Can you work these out from the model? Positions are in its coordinate system, mm. A direction names the side the tool comes from. Coordinates: 2 decimals unless noted, no trailing zeros. Write each loop counter-clockwise with the first axis right and the second up, starting at its lowest first coordinate (ties: lowest second). Pieces come first, ordered by that corner, then holes. Notation, with made-up numbers: M -36,1 L -3,1 A15 ccw -3,5 Z; hole C 70,-20.5 d8. An arc over 180 degrees is marked long. Use one line per item in the form item = value. Start each with the question number.
```python
from build123d import *

# Parameters (mm, degrees)
FILLET1_R                       = 2
BOSS_EXTRUDE1_REACH             = 54.062
SKETCH2_R                       = 1.5
BOSS_EXTRUDE1_DIRECTION_2_REACH = 54.062
CHAMFER1_SIZE                   = 1
CUT_EXTRUDE1_START              = -3
CUT_EXTRUDE1_DEPTH              = 3


with BuildPart() as part:
    # Sketch1 → Revolve1 (revolve)
    with BuildSketch(Plane.XY):
        Polygon((17.7, 0), (17.7, 3.5), (0, 28.778219719), (0, 43.98066929), (3, 43.98066929), (3, 27.98066929), (19.7, 4.130597578), (19.7, 0), align=None)
    revolve(axis=Axis((0, 0, 0), (0, 1, 0)))

    # Fillet1
    fillet1_edges = [part.edges().sort_by_distance(p)[0] for p in [
        (-3, 27.98066929, 0),
        (-19.7, 4.130597578, 0),
    ]]
    fillet(fillet1_edges, radius=FILLET1_R)

    # Boss-Extrude1: up to this cone (the profile starts inside it)
    boss_extrude1_end = Plane(origin=(0, 12, 0), z_dir=(0, -1, 0)).offset(-16.778218719) * Cone(1e-06, 58.179162981, 83.088454645, align=(Align.CENTER, Align.CENTER, Align.MIN), mode=Mode.PRIVATE)
    # Sketch2 → Boss-Extrude1 (add, up to the surface)
    with BuildSketch(Plane(origin=(0, 0, 0), x_dir=(0, 0, -1), z_dir=(1, 0, 0)), mode=Mode.PRIVATE) as boss_extrude1_sk1:
        with Locations(Location((0, 12, 0), (0, 0, 356.704943747))):
            Circle(SKETCH2_R)
    boss_extrude1_tool1 = extrude(boss_extrude1_sk1.sketch, amount=BOSS_EXTRUDE1_REACH, mode=Mode.PRIVATE) & boss_extrude1_end
    add(boss_extrude1_tool1.solids().sort_by_distance((0, 12, 0))[0])

    # Boss-Extrude1 direction 2: up to this cone (the profile starts inside it)
    boss_extrude1_direction_2_end = Plane(origin=(0, 12, 0), z_dir=(0, -1, 0)).offset(-16.778218719) * Cone(1e-06, 58.179162981, 83.088454645, align=(Align.CENTER, Align.CENTER, Align.MIN), mode=Mode.PRIVATE)
    # Sketch2 → Boss-Extrude1 direction 2 (add, up to the surface)
    with BuildSketch(Plane(origin=(0, 0, 0), x_dir=(0, 0, -1), z_dir=(1, 0, 0)), mode=Mode.PRIVATE) as boss_extrude1_direction_2_sk1:
        with Locations(Location((0, 12, 0), (0, 0, 356.704943747))):
            Circle(SKETCH2_R)
    boss_extrude1_direction_2_tool1 = extrude(boss_extrude1_direction_2_sk1.sketch, amount=-BOSS_EXTRUDE1_DIRECTION_2_REACH, mode=Mode.PRIVATE) & boss_extrude1_direction_2_end
    add(boss_extrude1_direction_2_tool1.solids().sort_by_distance((0, 12, 0))[0])

    # Chamfer1
    chamfer1_edges = [part.edges().sort_by_distance(p)[0] for p in [
        (-3, 43.98066929, 0),
    ]]
    chamfer(chamfer1_edges, length=CHAMFER1_SIZE)

    # Sketch3 → Cut-Extrude1 (cut)
    with BuildSketch(Plane.XZ.offset(CUT_EXTRUDE1_START)):
        with BuildLine():
            Line((-3.2, 18.627130751), (-3.2, 17.408331339))
            ThreePointArc((-3.2, 17.408331339), (0, 17.7), (3.2, 17.408331339))
            Line((3.2, 17.408331339), (3.2, 18.627130751))
            ThreePointArc((3.2, 18.627130751), (0, 18.9), (-3.2, 18.627130751))
        make_face()
        with BuildLine():
            Line((3.2, -17.408331339), (3.2, -18.627130751))
            ThreePointArc((3.2, -18.627130751), (0, -18.9), (-3.2, -18.627130751))
            Line((-3.2, -18.627130751), (-3.2, -17.408331339))
            ThreePointArc((-3.2, -17.408331339), (0, -17.7), (3.2, -17.408331339))
        make_face()
    extrude(amount=CUT_EXTRUDE1_DEPTH, mode=Mode.SUBTRACT)


solid = part.part
```
1) Suppose I cut it at B-B on y = 32. Please give me the cut outline in (x, z), and give its area (3 significant figures).
2) Suppose I cut it at A-A on y = 19. Please give me the cut outline in (x, z), and give its area (3 significant figures).
3) Will these pins go through, and if not, where does the flat tip stop? pin 1 Ø1.3 at (y, z) = (2, 18) entering from +X; pin 2 Ø12 at (x, z) = (15, 13) entering from +Y; pin 3 Ø5 at (x, z) = (-10.5, 9) entering from -Y.
4) If we mould it in two halves opening along Y, with no side actions, what happens to faces 1 (the face through (-18, 0, -3)), 2 (the face through (-0.18, 10.63, -0.61)), 3 (the face through (3.2, 2, -18))? For each: +Y half, -Y half, draft (parallel to the pull), parting line (faces both ways), or undercut.
5) Which directions (+Z, -Z, +X, -X, +Y, -Y) give clear straight access to the entire face, cutting with the end or side of a thin tool? Please do faces 4 (the face through (6.244, 19.125, 2.589)), 5 (the face through (0, 43.981, 0)), 6 (the face through (2.77, 35.7, 1.15)), 7 (the face through (0, 1.5, 18.9)).
6) Suppose I cut it at C-C on y = 7. Please give me the cut outline in (x, z), and give its area (3 significant figures).
7) Please list where these lines run through material, in increasing order: line 1 (X direction, y = 1.7, z = 0); line 2 (Z direction, x = 0, y = 2.2); line 3 (Z direction, x = -7.5, y = 12).
Computed values:
q1.outline = C 0,0 d6
q1.area = 28.3 mm²
q2.outline = C 0,0 d18.58; hole C 0,0 d13.69
q2.area = 124 mm²
q3.pin_1 = 9.33
q3.pin_2 = 12.49
q3.pin_3 = 5.46
q4.face_1 = -Y half
q4.face_2 = undercut
q4.face_3 = draft
q5.face_4 = none
q5.face_5 = +Z, -Z, +X, -X, +Y
q5.face_6 = +Y
q5.face_7 = -Y
q6.outline = C 0,0 d35.38; hole C 0,0 d30.5
q6.area = 253 mm²
q7.line_1 = -19.7 to -17.7, 17.7 to 19.7
q7.line_2 = -19.7 to -18.9, 18.9 to 19.7
q7.line_3 = -12.05 to -9.04, -1.5 to 1.5, 9.04 to 12.05
